from build123d import *

# Parameters (mm, degrees)
CUT_EXTRUDE8_DEPTH   = 3.5
SKETCH16_R           = 3.505318085
BOSS_EXTRUDE10_DEPTH = 0.2
SKETCH17_R           = 1.5
CUT_EXTRUDE9_DEPTH   = 5
CHAMFER2_SIZE        = 0.25


with BuildPart() as part:
    # Sketch6 → Revolve10 (revolve)
    with BuildSketch(Plane(origin=(0, 0, 0), x_dir=(1, 0, 0), z_dir=(0, 1, 0))):
        Polygon((9.015233675, -1.950120561), (9.015233675, -5.996890529), (6.215233675, -5.996890529), (6.215233675, -2.491572445), (6.527841066, -1.950120561), align=None)
    revolve(axis=Axis((5.148806832, 0, 5.996890529), (1, 0, 0)))

    # Sketch14 → Cut-Extrude8 (cut)
    with BuildSketch(Plane(origin=(9.015233675, 0, 0), x_dir=(0, 0, -1), z_dir=(1, 0, 0))):
        with BuildLine():
            Line((-8.020275514, 3.504605596), (-3.973505545, 3.504605596))
            ThreePointArc((-3.973505545, 3.504605596), (-5.996890529, 4.046769969), (-8.020275514, 3.504605596))
        make_face()
        with BuildLine():
            Line((-10.043660498, 0), (-8.020275514, 3.504605596))
            ThreePointArc((-8.020275514, 3.504605596), (-9.501496126, 2.023384984), (-10.043660498, 0))
        make_face()
        with BuildLine():
            ThreePointArc((-10.043660498, 0), (-9.501496126, -2.023384984), (-8.020275514, -3.504605596))
            Line((-8.020275514, -3.504605596), (-10.043660498, 0))
        make_face()
        with BuildLine():
            ThreePointArc((-8.020275514, -3.504605596), (-5.996890529, -4.046769969), (-3.973505545, -3.504605596))
            Line((-3.973505545, -3.504605596), (-8.020275514, -3.504605596))
        make_face()
        with BuildLine():
            ThreePointArc((-3.973505545, -3.504605596), (-2.492284933, -2.023384984), (-1.950120561, 0))
            Line((-1.950120561, 0), (-3.973505545, -3.504605596))
        make_face()
        with BuildLine():
            Line((-3.973505545, 3.504605596), (-1.950120561, 0))
            ThreePointArc((-1.950120561, 0), (-2.492284933, 2.023384984), (-3.973505545, 3.504605596))
        make_face()
    extrude(amount=-CUT_EXTRUDE8_DEPTH, mode=Mode.SUBTRACT)

    # Sketch16 → Boss-Extrude10 (add)
    with BuildSketch(Plane(origin=(9.015233675, 0, 0), x_dir=(0, 0, -1), z_dir=(1, 0, 0))):
        with Locations((-5.996890529, 0)):
            Circle(SKETCH16_R)
    extrude(amount=BOSS_EXTRUDE10_DEPTH)

    # Sketch17 → Cut-Extrude9 (cut)
    with BuildSketch(Plane(origin=(9.215233675, 0, 0), x_dir=(0, 0, -1), z_dir=(1, 0, 0))):
        with Locations((-5.996890529, 0)):
            Circle(SKETCH17_R)
    extrude(amount=-CUT_EXTRUDE9_DEPTH, mode=Mode.SUBTRACT)

    # Chamfer2
    chamfer2_edges = [part.edges().sort_by_distance(p)[0] for p in [
        (6.215233675, 0, 7.496890529),
        (9.215233675, 0, 7.496890529),
    ]]
    chamfer(chamfer2_edges, length=CHAMFER2_SIZE)


solid = part.part
Geometry check sheet. Reference: the model listing, model coordinates, mm. A direction names the side the tool comes from. Round coordinates to 2 decimals unless told otherwise and drop trailing zeros. Write each loop counter-clockwise with the first axis right and the second up, starting at its lowest first coordinate (ties: lowest second). Pieces come first, ordered by that corner, then holes.
Item 1: Material ranges on line 1 along Y through (x, z) = (6.95, 6.25); line 2 along Y through (x, z) = (8.2, 5); line 3 along X through (y, z) = (2.5, 3.5), recorded low to high.
Determined:
line 1: y = -3.5 to -1.48, 1.48 to 3.5
line 2: y = -3.5 to -1.12, 1.12 to 3.5
line 3: x = 6.23 to 9.02
Item 2: Section check A-A (x = 6.75). Record the boundary of the cut face in (y, z).
Determined:
outline: (-3.5, 3.97) - (0, 1.95) - (3.5, 3.97) - (3.5, 8.02) - (0, 10.04) - (-3.5, 8.02) - close; hole circle Ø3 at (0, 6)
Item 3: Mould release check, pull along Y, two halves, no side actions. Record for faces 6 (the face through (7.733, 0.066, 7.495)), 7 (the face through (7.635, -1.777, 9.018)), 8 (the face through (9.015, -0.1, 9.7)): +Y half, -Y half, draft (parallel to the pull), parting line (faces both ways), or undercut.
Determined:
face 6: undercut
face 7: -Y half
face 8: draft
Item 4: Access from +Z, -Z, +X, -X, +Y, -Y to the whole of each face (thin tool, end or side, straight path). Record for faces 1 (the face through (6.291, 0.009, 9.634)), 2 (the face through (9.015, 3.2, 4.1)), 3 (the face through (9.015, -3.2, 7.9)), 4 (the face through (9.015, 3.2, 7.8)), 5 (the face through (6.291, -3.154, 4.186)).
Determined:
face 1: +Z, -X
face 2: -Z, +X, +Y
face 3: +Z, +X, -Y
face 4: +Z, +X, +Y
face 5: -Z, -X, -Y
Item 5: Go/stop test with a flat-tipped pin: pin 1 Ø1.5 at (y, z) = (1, 5.5) entering from +X. Record where the tip stops, or that it passes through.
Determined:
pin 1: stops at x = 9.22
